```python
from build123d import *

# Parameters (mm, degrees)
SKETCH_1_R          = 13.7
EXTRUDE_1_DEPTH     = 2.3
SKETCH_2_R          = 12.49
EXTRUDE_2_DEPTH     = 7.7
SKETCH_3_R          = 5.01
SKETCH_3_R_2        = 1.65
CUT_EXTRUDE_1_DEPTH = 10


with BuildPart() as part:
    # ｽｹｯﾁ1 → ﾎﾞｽ - 押し出し1 (new body)
    with BuildSketch(Plane(origin=(0, 0, 0), x_dir=(1, 0, 0), z_dir=(0, 1, 0))):
        with Locations(Location((0, 0, 0), (0, 0, 270))):
            Circle(SKETCH_1_R)
    extrude(amount=EXTRUDE_1_DEPTH)

    # ｽｹｯﾁ2 → ﾎﾞｽ - 押し出し2 (add)
    with BuildSketch(Plane(origin=(0, 2.3, 0), x_dir=(1, 0, 0), z_dir=(0, 1, 0))):
        with Locations(Location((0, 0, 0), (0, 0, 270))):
            Circle(SKETCH_2_R)
    extrude(amount=EXTRUDE_2_DEPTH)

    # ｽｹｯﾁ3 → ｶｯﾄ - 押し出し1 (cut)
    with BuildSketch(Plane.XZ):
        with Locations(Location((0, 0, 0), (0, 0, 270))):
            Circle(SKETCH_3_R)
        with Locations(Location((9, 0, 0), (0, 0, 270))):
            Circle(SKETCH_3_R_2)
        with Locations(Location((-9, 0, 0), (0, 0, 90))):
            Circle(SKETCH_3_R_2)
    extrude(amount=-CUT_EXTRUDE_1_DEPTH, mode=Mode.SUBTRACT)


solid = part.part
```
Can you work these out from the model? Positions are in its coordinate system, mm. A direction names the side the tool comes from. Coordinates: 2 decimals unless noted, no trailing zeros. Write each loop counter-clockwise with the first axis right and the second up, starting at its lowest first coordinate (ties: lowest second). Pieces come first, ordered by that corner, then holes. Notation, with made-up numbers: M -28.75,41.5 L 30.25,41.5 A26 ccw 30.25,77.5 Z; hole C 84,-31 d11. An arc over 180 degrees is marked long. Answer as CSV lines item,"result".
Item 1: On a 3-axis mill with a long thin cutter (end or side, diameter ignored), from which of +Z, -Z, +X, -X, +Y, -Y can I reach the whole of each face in a straight line? I mean faces 5 (the flat face through (-4, 2.3, 12)), 6 (the cylindrical face through (4.115, 1.134, 13.067)). Say none if no direction works.
Geometry results:
face 5,"+Y"
face 6,"+Y, -Y"
Item 2: Imagine slicing it at B-B on x = 0. List the corners of the cut face in (y, z) for me.
Geometry results:
outline,"M 0,-13.7 L 2.3,-13.7 L 2.3,-12.49 L 10,-12.49 L 10,-5.01 L 0,-5.01 Z; M 0,5.01 L 10,5.01 L 10,12.49 L 2.3,12.49 L 2.3,13.7 L 0,13.7 Z"
Item 3: Imagine slicing it at A-A on z = 0. List the corners of the cut face in (x, y) for me.
Geometry results:
outline,"M -13.7,0 L -10.65,0 L -10.65,10 L -12.49,10 L -12.49,2.3 L -13.7,2.3 Z; M -7.35,0 L -5.01,0 L -5.01,10 L -7.35,10 Z; M 5.01,0 L 7.35,0 L 7.35,10 L 5.01,10 Z; M 10.65,0 L 13.7,0 L 13.7,2.3 L 12.49,2.3 L 12.49,10 L 10.65,10 Z"
Item 4: Imagine slicing it at D-D on z = 6.75. List the corners of the cut face in (x, y) for me.
Geometry results:
outline,"M -11.92,0 L 11.92,0 L 11.92,2.3 L 10.51,2.3 L 10.51,10 L -10.51,10 L -10.51,2.3 L -11.92,2.3 Z"
Item 5: Please list where these lines run through material, in increasing order: line 1 along X through (y, z) = (2.75, 0); line 2 along X through (y, z) = (6, 1.5); line 3 along Y through (x, z) = (-7, -11.5).
Geometry results:
line 1,"x = -12.49 to -10.65, -7.35 to -5.01, 5.01 to 7.35, 10.65 to 12.49"
line 2,"x = -12.4 to -9.69, -8.31 to -4.78, 4.78 to 8.31, 9.69 to 12.4"
line 3,"y = 0 to 2.3"
Item 6: We'd pull the mould along X, two halves only. Please class faces 1 (the cylindrical face through (-7.4, 4.9, -0.4)), 2 (the cylindrical face through (1.5, 4.93, -4.78)), 3 (the cylindrical face through (10.532, 6.096, 6.715)), 4 (the flat face through (0, 0, 6)): +X half, -X half, draft (parallel to the pull), parting line (faces both ways), or undercut.
Geometry results:
face 1,"undercut"
face 2,"undercut"
face 3,"parting line"
face 4,"draft"
Item 7: Imagine slicing it at C-C on y = 1.5. List the corners of the cut face in (x, z) for me.
Geometry results:
outline,"C 0,0 d27.4; hole C -9,0 d3.3; hole C 0,0 d10.02; hole C 9,0 d3.3"
Item 8: I'm going to push flat-ended pins straight in: P1, Ø6, axis at x = 0, z = 0, coming from the -Y side; P2, Ø5, axis at x = -11, y = 2.5, coming from the +Z side; P3, Ø2, axis at x = -10, y = 3, coming from the +Z side. Where does each tip first touch, or does it pass through?
Geometry results:
P1,"passes through"
P2,"stops at z = 10.74"
P3,"stops at z = 10.07"
